Design review of the part built by this model. Coordinates are the model's own, in mm. A direction names the side the tool comes from. Coordinates: 2 decimals unless noted, no trailing zeros. Loops run counter-clockwise (first coordinate to the right, second up) from the corner with the lowest first, then second, coordinate; pieces in that order, holes last. Notation, with made-up numbers: M 22.5,54.5 L 61.5,54.5 A18 ccw 61.5,62.5 Z; hole C -24.75,63.25 d9. An arc over 180 degrees is marked long. Answer as CSV lines item,"result". Start each with the question number.
Autodesk Inventor part; units mm, degrees
ref_plane "YZ Plane" through (0, 0, 0) normal (1, 0, 0) x (0, 1, 0)
ref_plane "XZ Plane" through (0, 0, 0) normal (0, 1, 0) x (-1, 0, 0)
ref_plane "XY Plane" through (0, 0, 0) normal (0, 0, 1) x (1, 0, 0)
sketch "Sketch1" plane through (0, 0, 0) normal (0, 0, 1) x (1, 0, 0)
  circle A0 centre (-48.56, 6.9152) radius 2.1
  circle A1 centre (-32.9741, 22.501) radius 2.1
  circle A2 centre (-69.0444, -1.2227) radius 2.1
  circle A3 centre (-24.8362, 42.9855) radius 2.1
  circle A4 centre (-46.3856, -8.3913) radius 8
  line L0 (-28.6687, 48.4472) -> (-17.4995, 54.7179)
  arc A5 (-69.8258, 3.2089) -> (-28.6687, 48.4472) centre (-78.5082, 52.4493) ccw
  line L1 (-69.8258, 3.2089) -> (-78.128, 1.745)
  line L2 (-78.128, 1.745) -> (-74.0482, -21.3924)
  line L3 (-74.0482, -21.3924) -> (-70.3922, -20.7477)
  arc A6 (-70.3922, -20.7477) -> (-49.7861, -35.1763) centre (-46.3856, -8.3913) ccw
  line L4 (-49.7861, -35.1763) -> (-49.1414, -38.8323)
  line L5 (-49.1414, -38.8323) -> (-41.263, -37.4431)
  line L6 (-41.263, -37.4431) -> (4.3164, -53.3072)
  line L7 (4.3164, -53.3072) -> (1.8974, -59.9532)
  line L8 (1.8974, -59.9532) -> (17.5702, -63.2237)
  arc A7 (17.5702, -63.2237) -> (22.7521, -63.408) centre (22.2724, -3.9734) ccw
  line L9 (22.7521, -63.408) -> (22.7442, -62.4373)
  arc A8 (24.6597, -60.4229) -> (22.7442, -62.4373) centre (24.7442, -62.4211) ccw
  arc A9 (24.6597, -60.4229) -> (33.3265, -59.3815) centre (22.2724, -3.9734) ccw
  arc A10 (35.6646, -60.8847) -> (33.3265, -59.3815) centre (33.7178, -61.3428) ccw
  line L10 (35.6646, -60.8847) -> (35.9706, -62.1851)
  arc A11 (35.9706, -62.1851) -> (41.9803, -60.4344) centre (22.2724, -3.9734) ccw
  line L11 (41.9803, -60.4344) -> (52.856, -55.363)
  arc A12 (52.856, -55.363) -> (58.0602, -51.8846) centre (22.2724, -3.9734) ccw
  line L12 (58.0602, -51.8846) -> (57.2607, -50.8143)
  arc A13 (57.6121, -48.0569) -> (57.2607, -50.8143) centre (58.863, -49.6174) ccw
  arc A14 (57.6121, -48.0569) -> (63.9808, -42.0872) centre (22.2724, -3.9734) ccw
  arc A15 (66.7551, -41.9147) -> (63.9808, -42.0872) centre (65.4572, -43.4363) ccw
  line L13 (66.7551, -41.9147) -> (67.4937, -42.5447)
  arc A16 (67.4937, -42.5447) -> (70.6833, -38.4566) centre (22.2724, -3.9734) ccw
  line L14 (70.6833, -38.4566) -> (78.2523, -24.3484)
  line L15 (78.2523, -24.3484) -> (71.6063, -21.9294)
  arc A17 (71.6063, -21.9294) -> (67.7387, 22.2766) centre (22.2724, -3.9734) ccw
  line L16 (67.7387, 22.2766) -> (73.8637, 25.8129)
  line L17 (73.8637, 25.8129) -> (63.9599, 38.3925)
  arc A18 (63.9599, 38.3925) -> (60.1088, 41.8646) centre (22.2724, -3.9734) ccw
  line L18 (60.1088, 41.8646) -> (59.4908, 41.1159)
  arc A19 (56.7287, 40.804) -> (59.4908, 41.1159) centre (57.9484, 42.389) ccw
  arc A20 (56.7287, 40.804) -> (49.4201, 45.5771) centre (22.2724, -3.9734) ccw
  arc A21 (48.5953, 48.2316) -> (49.4201, 45.5771) centre (50.3811, 47.3311) ccw
  line L19 (48.5953, 48.2316) -> (49.1968, 49.4245)
  arc A22 (49.1968, 49.4245) -> (43.4677, 51.9463) centre (22.2724, -3.9734) ccw
  line L20 (43.4677, 51.9463) -> (31.8766, 55.0521)
  arc A23 (31.8766, 55.0521) -> (25.6541, 55.7327) centre (22.2724, -3.9734) ccw
  line L21 (25.6541, 55.7327) -> (25.5786, 54.3989)
  arc A24 (23.537, 52.5125) -> (25.5786, 54.3989) centre (23.5818, 54.512) ccw
  arc A25 (23.537, 52.5125) -> (14.821, 52.0331) centre (22.2724, -3.9734) ccw
  arc A26 (12.5849, 53.6843) -> (14.821, 52.0331) centre (14.5573, 54.0157) ccw
  line L22 (12.5849, 53.6843) -> (12.4241, 54.6417)
  arc A27 (12.4241, 54.6417) -> (7.3529, 53.5603) centre (22.2724, -3.9734) ccw
  line L23 (7.3529, 53.5603) -> (-7.5139, 47.618)
  line L24 (-7.5139, 47.618) -> (-17.4995, 54.7179)
  circle A28 centre (-71.296, -16.8454) radius 1.5
  circle A29 centre (18.8152, -59.8032) radius 1.5
  circle A30 centre (53.4562, -50.8504) radius 1.5
  circle A31 centre (60.8075, 36.5725) radius 1.5
  circle A32 centre (28.5162, 51.9811) radius 1.5
  circle A33 centre (9.173, 50.4079) radius 1.5
  circle A34 centre (44.8423, 47.6065) radius 1.5
  circle A35 centre (67.2628, -37.2117) radius 1.5
  circle A36 centre (38.1378, -57.9935) radius 1.5
  circle A37 centre (-45.81, -34.6909) radius 1.5
  circle A38 centre (22.2724, -3.9734) radius 32.5
  circle A39 centre (-78.5082, 52.4493) radius 5.9
  circle A40 centre (-78.5082, 52.4493) radius 50
  circle A41 centre (-78.5082, 52.4493) radius 54
  line L25 (-78.5082, 52.4493) -> (-69.0444, -1.2227)
  line L26 (-78.5082, 52.4493) -> (-24.8362, 42.9855)
  point P0 (0, 0)
  point P1 (-25.3286, 43.0723)
  point P2 (-29.2678, 43.7669)
  point P3 (-69.1312, -0.7303)
  dimension "d0" = 100
  dimension "d1" = 108
extrude "Extrusion1" add sketch "Sketch1" along normal blind 7.3 contours A41 A0 | A0 A41 A2 L25 A5 L26 A3 A1 | A1 A41 | A41 L25 A2 | A3 L26 A41 picked at (-49.1962, 7.731) picked at (-33.8814, 22.9981) picked at (-68.8495, -0.1546) picked at (-25.9043, 42.7906)
sketch "Sketch2" plane through (0, 0, 7.3) normal (0, 0, 1) x (1, 0, 0)
  circle A0 centre (-48.56, 6.9152) radius 2.1
  circle A1 centre (-32.9741, 22.501) radius 2.1
  circle A2 centre (-69.0444, -1.2227) radius 2.1
  circle A3 centre (-24.8362, 42.9855) radius 2.1
  circle A4 centre (-46.3856, -8.3913) radius 8
  line L0 (-28.6687, 48.4472) -> (-17.4995, 54.7179)
  arc A5 (-69.8258, 3.2089) -> (-28.6687, 48.4472) centre (-78.5082, 52.4493) ccw
  line L1 (-69.8258, 3.2089) -> (-78.128, 1.745)
  line L2 (-78.128, 1.745) -> (-74.0482, -21.3924)
  line L3 (-74.0482, -21.3924) -> (-70.3922, -20.7477)
  arc A6 (-70.3922, -20.7477) -> (-49.7861, -35.1763) centre (-46.3856, -8.3913) ccw
  line L4 (-49.7861, -35.1763) -> (-49.1414, -38.8323)
  line L5 (-49.1414, -38.8323) -> (-41.263, -37.4431)
  line L6 (-41.263, -37.4431) -> (4.3164, -53.3072)
  line L7 (4.3164, -53.3072) -> (1.8974, -59.9532)
  line L8 (1.8974, -59.9532) -> (17.5702, -63.2237)
  arc A7 (17.5702, -63.2237) -> (22.7521, -63.408) centre (22.2724, -3.9734) ccw
  line L9 (22.7521, -63.408) -> (22.7442, -62.4373)
  arc A8 (24.6597, -60.4229) -> (22.7442, -62.4373) centre (24.7442, -62.4211) ccw
  arc A9 (24.6597, -60.4229) -> (33.3265, -59.3815) centre (22.2724, -3.9734) ccw
  arc A10 (35.6646, -60.8847) -> (33.3265, -59.3815) centre (33.7178, -61.3428) ccw
  line L10 (35.6646, -60.8847) -> (35.9706, -62.1851)
  arc A11 (35.9706, -62.1851) -> (41.9803, -60.4344) centre (22.2724, -3.9734) ccw
  line L11 (41.9803, -60.4344) -> (52.856, -55.363)
  arc A12 (52.856, -55.363) -> (58.0602, -51.8846) centre (22.2724, -3.9734) ccw
  line L12 (58.0602, -51.8846) -> (57.2607, -50.8143)
  arc A13 (57.6121, -48.0569) -> (57.2607, -50.8143) centre (58.863, -49.6174) ccw
  arc A14 (57.6121, -48.0569) -> (63.9808, -42.0872) centre (22.2724, -3.9734) ccw
  arc A15 (66.7551, -41.9147) -> (63.9808, -42.0872) centre (65.4572, -43.4363) ccw
  line L13 (66.7551, -41.9147) -> (67.4937, -42.5447)
  arc A16 (67.4937, -42.5447) -> (70.6833, -38.4566) centre (22.2724, -3.9734) ccw
  line L14 (70.6833, -38.4566) -> (78.2523, -24.3484)
  line L15 (78.2523, -24.3484) -> (71.6063, -21.9294)
  arc A17 (71.6063, -21.9294) -> (67.7387, 22.2766) centre (22.2724, -3.9734) ccw
  line L16 (67.7387, 22.2766) -> (73.8637, 25.8129)
  line L17 (73.8637, 25.8129) -> (63.9599, 38.3925)
  arc A18 (63.9599, 38.3925) -> (60.1088, 41.8646) centre (22.2724, -3.9734) ccw
  line L18 (60.1088, 41.8646) -> (59.4908, 41.1159)
  arc A19 (56.7287, 40.804) -> (59.4908, 41.1159) centre (57.9484, 42.389) ccw
  arc A20 (56.7287, 40.804) -> (49.4201, 45.5771) centre (22.2724, -3.9734) ccw
  arc A21 (48.5953, 48.2316) -> (49.4201, 45.5771) centre (50.3811, 47.3311) ccw
  line L19 (48.5953, 48.2316) -> (49.1968, 49.4245)
  arc A22 (49.1968, 49.4245) -> (43.4677, 51.9463) centre (22.2724, -3.9734) ccw
  line L20 (43.4677, 51.9463) -> (31.8766, 55.0521)
  arc A23 (31.8766, 55.0521) -> (25.6541, 55.7327) centre (22.2724, -3.9734) ccw
  line L21 (25.6541, 55.7327) -> (25.5786, 54.3989)
  arc A24 (23.537, 52.5125) -> (25.5786, 54.3989) centre (23.5818, 54.512) ccw
  arc A25 (23.537, 52.5125) -> (14.821, 52.0331) centre (22.2724, -3.9734) ccw
  arc A26 (12.5849, 53.6843) -> (14.821, 52.0331) centre (14.5573, 54.0157) ccw
  line L22 (12.5849, 53.6843) -> (12.4241, 54.6417)
  arc A27 (12.4241, 54.6417) -> (7.3529, 53.5603) centre (22.2724, -3.9734) ccw
  line L23 (7.3529, 53.5603) -> (-7.5139, 47.618)
  line L24 (-7.5139, 47.618) -> (-17.4995, 54.7179)
  circle A28 centre (-71.296, -16.8454) radius 1.5
  circle A29 centre (18.8152, -59.8032) radius 1.5
  circle A30 centre (53.4562, -50.8504) radius 1.5
  circle A31 centre (60.8075, 36.5725) radius 1.5
  circle A32 centre (28.5162, 51.9811) radius 1.5
  circle A33 centre (9.173, 50.4079) radius 1.5
  circle A34 centre (44.8423, 47.6065) radius 1.5
  circle A35 centre (67.2628, -37.2117) radius 1.5
  circle A36 centre (38.1378, -57.9935) radius 1.5
  circle A37 centre (-45.81, -34.6909) radius 1.5
  circle A38 centre (22.2724, -3.9734) radius 32.5
  line L25 (-78.5082, 52.4493) -> (-69.0444, -1.2227)
  line L26 (-64.4974, -3.975) -> (-72.3759, -5.3642)
  line L27 (-72.3759, -5.3642) -> (-73.5914, 1.5295)
  line L28 (-73.5914, 1.5295) -> (-65.7129, 2.9187)
  line L29 (-65.7129, 2.9187) -> (-64.4974, -3.975)
  line L30 (-64.4974, -3.975) -> (-73.5914, 1.5295) construction
  line L31 (-72.3759, -5.3642) -> (-65.7129, 2.9187) construction
  line L32 (-43.2948, 6.189) -> (-49.9787, 1.793)
  line L33 (-47.1413, 12.0374) -> (-43.2948, 6.189)
  line L34 (-53.8252, 7.6414) -> (-47.1413, 12.0374)
  line L35 (-49.9787, 1.793) -> (-53.8252, 7.6414)
  line L36 (-27.8519, 23.9197) -> (-32.248, 17.2358)
  line L37 (-33.7003, 27.7663) -> (-27.8519, 23.9197)
  line L38 (-38.0964, 21.0824) -> (-33.7003, 27.7663)
  line L39 (-32.248, 17.2358) -> (-38.0964, 21.0824)
  line L40 (-20.6948, 46.3169) -> (-22.084, 38.4385)
  line L41 (-27.5884, 47.5325) -> (-20.6948, 46.3169)
  line L42 (-28.9776, 39.654) -> (-27.5884, 47.5325)
  line L43 (-22.084, 38.4385) -> (-28.9776, 39.654)
  line L44 (-72.3759, -5.3642) -> (-76.7388, -6.1335)
  line L45 (-28.6687, 48.4472) -> (-20.5709, 47.0193)
  line L46 (-20.5709, 47.0193) -> (-20.6948, 46.3169)
  line L47 (-25.3286, 43.0723) -> (-29.2678, 43.7669)
  point P0 (0, 0)
  point P1 (-69.6522, 2.2241)
  point P2 (-28.283, 43.5932)
  dimension "d4" = 8
  dimension "d5" = 7
  dimension "d8" = 70
extrude "Extrusion2" add sketch "Sketch2" against normal blind 7.3 contours A0 | A1 | A2 | L28 L29 L26 L27 | L28 L27 L44 L2 L1 L25 | A5 L45 L46 L41 L42 L47 | L42 L41 L40 L43 | A3 | L32 L35 L34 L33 | L36 L39 L38 L37
sketch "Sketch3" plane through (0, 0, 7.3) normal (0, 0, 1) x (1, 0, 0)
  circle A0 centre (-24.8362, 42.9855) radius 2.1
  circle A1 centre (-32.9741, 22.501) radius 2.1
  circle A2 centre (-48.56, 6.9152) radius 2.1
  circle A3 centre (-69.0444, -1.2227) radius 2.1
  point P0 (0, 0)
hole "Hole1" at (-24.8362, 42.9855, 7.3) at (-32.9741, 22.501, 7.3) at (-48.56, 6.9152, 7.3) at (-69.0444, -1.2227, 7.3) direction (0, 0, -1) diameter 3.1 depth 17
fillet "Fillet1" radius 2 6 edges at (-65.2178, 0.1104, 3.65) (-52.2582, 5.2588, 3.65) (-45.5743, 9.6549, 3.65) (-35.7139, 19.5154, 3.65) (-31.3178, 26.1993, 3.65) (-26.1693, 39.1588, 3.65)
properties part number "shell_5" material "ABS Plastic"
Item 1: For line 1 along Y through (x, z) = (-48.56, 5.75); line 2 along X through (y, z) = (7, 2.5); line 3 along X through (y, z) = (42, 3), list the stretches that pass through material, from the lowest coordinate up. Write a range as from..to.
Item 2: Add section B-B (z = 6.5). Give the number of separate pieces and of enclosed holes in the cut face, plus the area to 3 significant figures.
Item 3: For pin 1 (1.9 mm diameter, centred on x = -69.04, y = -1.22, fed in from -Z); pin 2 (1.5 mm diameter, centred on y = 40, z = 3.5, fed in from -X); pin 3 (4 mm diameter, centred on y = 7.5, z = 2.5, fed in from +X), all flat-tipped, find the tip position at first contact; note any pin that passes through.
Item 4: Add section C-C (y = 36). Give the boundary of the cut face in (x, z).
Item 5: Add section D-D (x = -62.5). Give the boundary of the cut face in (y, z).
Item 6: For faces 1 (the face through (-23.212, 38.637, 3.701)), 2 (the face through (-64.7, -2.82, 3.7)), 3 (the face through (-46.59, 4.02, 3.7)), list the 3-axis set-ups (+Z, -Z, +X, -X, +Y, -Y) from which the entire face can be reached by the end or side of a thin tool; tool diameter is ignored.
Item 7: Mouldability with a two-part tool opening along X and no side actions: class faces 4 (the face through (-30.02, 20.62, 3.7)), 5 (the face through (-33.04, 24.05, 3.6)), 6 (the face through (-47, 13, 0)) as released by +X, released by -X, zero draft, split by the parting line, or undercut.
Item 8: Add section A-A (x = -48.56). Give the boundary of the cut face in (y, z), plus the area to 3 significant figures.
Response:
1,line 1,"2.73..5.37, 8.47..12.41"
1,line 2,"-57.67..-50.11, -47.01..-43.83"
1,line 3,"-29.61..-26.03, -23.64..-21.46"
2,separate pieces,"1"
2,enclosed holes,"4"
2,area,"431 mm²"
3,pin 1,"through"
3,pin 2,"x = -30.28"
3,pin 3,"x = -43.29"
4,outline,"M -31.29,0 L -27.07,0 L -27.07,7.3 L -31.29,7.3 Z"
5,outline,"M 0.88,0 L 5.08,0 L 5.08,7.3 L 0.88,7.3 Z"
6,face 1,"+Z, -Z, -Y"
6,face 2,"+Z, -Z, +X"
6,face 3,"+Z, -Z, +X, -Y"
7,face 4,"released by +X"
7,face 5,"undercut"
7,face 6,"zero draft"
8,outline,"M 2.73,0 L 5.37,0 L 5.37,7.3 L 2.73,7.3 Z; M 8.47,0 L 12.41,0 L 12.41,7.3 L 8.47,7.3 Z"
8,area,"48.1 mm²"
